For this review, use the dimensioned drawing (mm, ordinates from the lowest corner) and the shaded views. A direction names the side the tool comes from. Round coordinates to 2 decimals unless told otherwise and drop trailing zeros. Write each loop counter-clockwise with the first axis right and the second up, starting at its lowest first coordinate (ties: lowest second). Pieces come first, ordered by that corner, then holes. Notation, with made-up numbers: M 50.5,14.25 L 88.5,14.25 A14 cw 88.5,18.25 Z; hole C -5.5,0 d9. An arc over 180 degrees is marked long. Write each question's results on one line, items separated by ' | '. Start each with the question number.
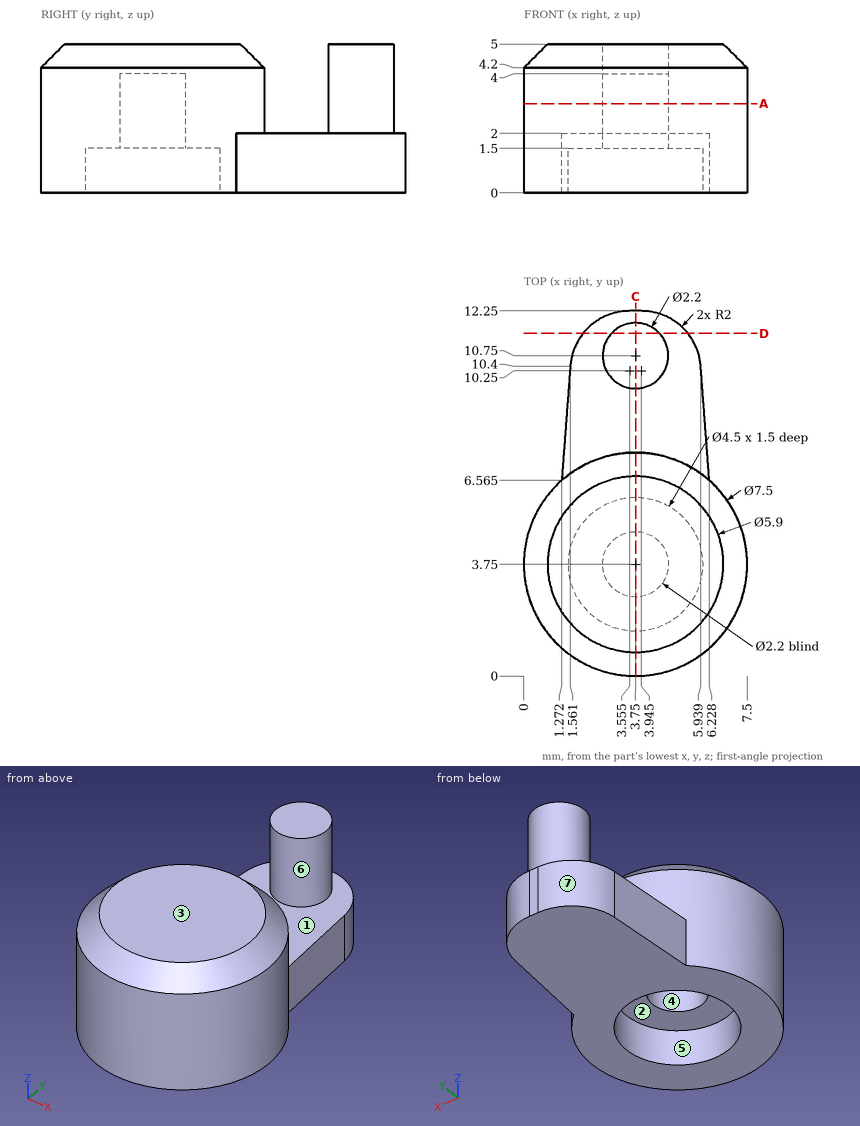
Item 1: We need section D-D on y = 11.5. State the section outline as (x, z) points (1 decimal).
Item 2: For the marked faces 1, 2 and 3, list the 3-axis set-ups (+Z, -Z, +X, -X, +Y, -Y) from which the entire face can be reached by the end or side of a thin tool; tool diameter is ignored.
Item 3: For probe 1 along Y at (x, z) = (3.75, 3.2); probe 2 along Y at (x, z) = (4.25, 3.75) (1 decimal); probe 3 along X at (y, z) = (5.25, 1) (1 decimal), list the stretches that pass through material, from the lowest coordinate up.
Item 4: We need section A-A on z = 3. State how many separate pieces and enclosed holes the cut face has.
Item 5: We need section C-C on x = 3.75. State the section outline as (y, z) points, then the cut area to 3 significant figures.
Item 6: Mouldability with a two-part tool opening along X and no side actions: class the marked faces 4, 5, 6 and 7 as pulls with the +X half, pulls with the -X half, needs draft (parallel to the pull), parting line crosses it, or undercut.
Item 7: Insertion check: P1, Ø2.5, axis at x = 3.75, y = 3.75, coming from the -Z side; P2, Ø2, axis at x = 3.5, z = 4.5, coming from the +Y side; P3, Ø3, axis at x = 1, z = 1, coming from the +Y side. Each pin has a flat end and moves straight along its axis. Give the tip position at first contact, or say it passes through.
Numbers:
1) outline: M 2,0 L 5.5,0 L 5.5,2 L 4.6,2 L 4.6,5 L 2.9,5 L 2.9,2 L 2,2 Z
2) face 1: +Z | face 2: -Z | face 3: +Z, +X, -X, +Y, -Y
3) probe 1: y = 0 to 2.65, 4.85 to 7.5, 9.65 to 11.85 | probe 2: y = 0 to 2.8, 4.7 to 7.5, 9.8 to 11.7 | probe 3: x = 0.3 to 2.1, 5.4 to 7.2
4) separate pieces: 2 | enclosed holes: 1
5) outline: M 0,0 L 1.5,0 L 1.5,1.5 L 2.65,1.5 L 2.65,4 L 4.85,4 L 4.85,1.5 L 6,1.5 L 6,0 L 12.25,0 L 12.25,2 L 11.85,2 L 11.85,5 L 9.65,5 L 9.65,2 L 7.5,2 L 7.5,4.2 L 6.7,5 L 0.8,5 L 0,4.2 Z | area: 40.7 mm^2
6) face 4: undercut | face 5: undercut | face 6: parting line crosses it | face 7: pulls with the -X half
7) P1: stops at z = 1.5 | P2: stops at y = 11.85 | P3: stops at y = 11.95
